The model under review builds one solid part; all positions refer to its coordinate system, in mm. A direction names the side the tool comes from. Round coordinates to 2 decimals unless told otherwise and drop trailing zeros. Write each loop counter-clockwise with the first axis right and the second up, starting at its lowest first coordinate (ties: lowest second). Pieces come first, ordered by that corner, then holes. Notation, with made-up numbers: (-12.75, -37) -> (34.25, -37) arc R31 ccw to (34.25, -1) -> close; hole circle Ø10 at (-3.5, 84.25). An arc over 180 degrees is marked (long way). Answer as a JSON object with one key per item and string values. Group by question number.
1) We need section A-A, the plane y = 0. Write out the cut boundary in (x, z).
2) Insertion check: pin 1 Ø1.5 at (x, z) = (5, 50.5) entering from -Y; pin 2 Ø12 at (y, z) = (2.5, 33.5) entering from +X; pin 3 Ø12 at (x, y) = (8.5, -5.5) entering from -Z; pin 4 Ø5 at (y, z) = (-5, 54.5) entering from +X. Each pin has a flat end and moves straight along its axis. Give the tip position at first contact, or say it passes through.
3) To check wall thickness, follow probe 1 along X at (y, z) = (0.5, 202.5); probe 2 along Z at (x, y) = (-8.25, 3.25); probe 3 along Y at (x, z) = (-0.75, 51.5). State the ranges of each line that lie inside material, in increasing order. Write a range as [from, to].
4) We need section C-C, the plane z = 176.5. Write out the cut boundary in (x, y).
5) We need section B-B, the plane x = 2.25. Write out the cut boundary in (y, z).
6) Machinability: for faces 1 (the flat face through (-2.909, -5.133, 222.606)), 2 (the flat face through (-2.991, 5.086, 222.606)), 3 (the flat face through (2.991, -5.086, 222.606)), 4 (the flat face through (2.909, 5.133, 222.606)), 5 (the flat face through (5.9, 0, 223)), which of the approach directions +Z, -Z, +X, -X, +Y, -Y give a long, thin tool a straight path to every point of the face, cutting with its end or side? Answer none if there is none.
7) We need section D-D, the plane x = -8.5. Write out the cut boundary in (y, z), then the cut area to 3 significant figures.
Autodesk Inventor part; units mm, degrees
ref_plane "YZ Plane" through (0, 0, 0) normal (1, 0, 0) x (0, 1, 0)
ref_plane "XZ Plane" through (0, 0, 0) normal (0, 1, 0) x (-1, 0, 0)
ref_plane "XY Plane" through (0, 0, 0) normal (0, 0, 1) x (1, 0, 0)
sketch "スケッチ1" plane through (0, 0, 0) normal (0, 0, 1) x (1, 0, 0)
  circle A0 centre (0, 0) radius 5.95
  dimension "d0" = 11.9
extrude "押し出し1" add sketch "スケッチ1" along normal blind 215
thread "ねじ1"
sketch "スケッチ2" plane through (0, 0, 215) normal (0, 0, 1) x (1, 0, 0)
  circle A0 centre (0, 0) radius 11.3
  dimension "d5" = 22.6
extrude "押し出し2" add sketch "スケッチ2" along normal blind 4.5
sketch "スケッチ3" plane through (0, 0, 219.5) normal (0, 0, 1) x (1, 0, 0)
  circle A0 centre (0, 0) radius 5.9 construction
  line L0 (5.9, -3.4064) -> (0, -6.8127)
  line L1 (0, -6.8127) -> (-5.9, -3.4064)
  line L2 (-5.9, -3.4064) -> (-5.9, 3.4064)
  line L3 (-5.9, 3.4064) -> (0, 6.8127)
  line L4 (0, 6.8127) -> (5.9, 3.4064)
  line L5 (5.9, 3.4064) -> (5.9, -3.4064)
  point P0 (5.9, 0)
  dimension "d8" = 11.8
extrude "押し出し3" add sketch "スケッチ3" along normal blind 6.3
properties part number "後輪シャフト"
Here are the results:
{
 "1": {"outline": "(-11.3, 215) -> (-5.95, 215) -> (-5.95, 0) -> (5.95, 0) -> (5.95, 215) -> (11.3, 215) -> (11.3, 219.5) -> (5.9, 219.5) -> (5.9, 225.8) -> (-5.9, 225.8) -> (-5.9, 219.5) -> (-11.3, 219.5) -> close"},
 "2": {"pin 1": "stops at y = -4.16", "pin 2": "stops at x = 5.95", "pin 3": "stops at z = 0", "pin 4": "stops at x = 5.4"},
 "3": {"probe 1": "x = [-5.93, 5.93]", "probe 2": "z = [215, 219.5]", "probe 3": "y = [-5.9, 5.9]"},
 "4": {"outline": "circle Ø11.9 at (0, 0)"},
 "5": {"outline": "(-11.07, 215) -> (-5.51, 215) -> (-5.51, 0) -> (5.51, 0) -> (5.51, 215) -> (11.07, 215) -> (11.07, 219.5) -> (5.51, 219.5) -> (5.51, 225.8) -> (-5.51, 225.8) -> (-5.51, 219.5) -> (-11.07, 219.5) -> close"},
 "6": {"face 1": "+Z, -X, -Y", "face 2": "+Z, -X, +Y", "face 3": "+Z, +X, -Y", "face 4": "+Z, +X, +Y", "face 5": "+Z, +X, +Y, -Y"},
 "7": {"outline": "(-7.45, 215) -> (7.45, 215) -> (7.45, 219.5) -> (-7.45, 219.5) -> close", "area": "67.0 mm^2"}
}
